The model under review builds one solid part; all positions refer to its coordinate system, in mm. A direction names the side the tool comes from. Give positions to 0.01 mm unless a question says otherwise; leave off trailing zeros. Loops run counter-clockwise (first coordinate to the right, second up) from the corner with the lowest first, then second, coordinate; pieces in that order, holes last. Notation, with made-up numbers: (27, -36) - (73, -36) arc R18 cw to (73, -23) - close; hole circle Ø10 at (33.5, -16). An arc over 180 degrees is marked (long way). Return JSON: item names as keys, results as strings. Group by question number.
```python
from build123d import *

# Parameters (mm, degrees)
EXTRUDE_START       = 2
SKETCH_3_R          = 40.25
SKETCH_3_R_2        = 1.6
SKETCH_3_R_3        = 17.5
EXTRUDE_1_DEPTH     = 3
SKETCH_3_4_R        = 17.5
SKETCH_3_4_R_2      = 2.1
EXTRUDE_3_DEPTH     = 2.5
CHAMFER_1_SIZE      = 3
CHAMFER_4_SIZE      = 2.5
SKETCH_4_R          = 40.25
SKETCH_4_R_2        = 33
SKETCH_4_R_3        = 1.6
EXTRUDE_4_DEPTH     = 2
CUT_EXTRUDE_START   = -13
SKETCH_4_4_R        = 40.25
SKETCH_4_4_R_2      = 33
SKETCH_4_4_R_3      = 1.6
CUT_EXTRUDE_4_DEPTH = 12
CHAMFER_5_SIZE      = 2
CHAMFER_8_SIZE      = 2
SKETCH_5_R          = 1.6
EXTRUDE_5_DEPTH     = 6.5


# Some blends are built 0.0001 mm under size
with BuildPart() as part:
    # 草图3 → 凸台-拉伸1 (new body)
    with BuildSketch(Plane(origin=(0, 0, 0), x_dir=(1, 0, 0), z_dir=(0, 1, 0)).offset(EXTRUDE_START)):
        with Locations(Location((-0.44726781, 0.687620087, 0), (0, 0, 270))):
            Circle(SKETCH_3_R)
        with Locations(Location((-15.663111428, 34.961926834, 0), (0, 0, 270))):
            Circle(SKETCH_3_R_2, mode=Mode.SUBTRACT)
        with Locations(Location((9.927819446, 36.723818061, 0), (0, 0, 270))):
            Circle(SKETCH_3_R_2, mode=Mode.SUBTRACT)
        with Locations(Location((30.664131688, 21.623971758, 0), (0, 0, 270))):
            Circle(SKETCH_3_R_2, mode=Mode.SUBTRACT)
        with Locations(Location((36.843074339, -3.272226173, 0), (0, 0, 270))):
            Circle(SKETCH_3_R_2, mode=Mode.SUBTRACT)
        with Locations(Location((25.573451463, -26.315568031, 0), (0, 0, 270))):
            Circle(SKETCH_3_R_2, mode=Mode.SUBTRACT)
        with Locations(Location((2.128444851, -36.723818061, 0), (0, 0, 270))):
            Circle(SKETCH_3_R_2, mode=Mode.SUBTRACT)
        with Locations(Location((-22.521766341, -29.6268404, 0), (0, 0, 270))):
            Circle(SKETCH_3_R_2, mode=Mode.SUBTRACT)
        with Locations(Location((-36.843074339, -8.34538977, 0), (0, 0, 270))):
            Circle(SKETCH_3_R_2, mode=Mode.SUBTRACT)
        with Locations(Location((-34.134379969, 17.162706563, 0), (0, 0, 270))):
            Circle(SKETCH_3_R_2, mode=Mode.SUBTRACT)
        with Locations(Location((-0.44726781, 0.687620087, 0), (0, 0, 270))):
            Circle(SKETCH_3_R_3, mode=Mode.SUBTRACT)
    extrude(amount=EXTRUDE_1_DEPTH)

    # 草图3<4> → 凸台-拉伸3 (add)
    with BuildSketch(Plane(origin=(0, 0, 0), x_dir=(1, 0, 0), z_dir=(0, 1, 0))):
        with Locations(Location((-0.44726781, 0.687620087, 0), (0, 0, 270))):
            Circle(SKETCH_3_4_R)
        with Locations(Location((-1.271495861, 12.659280294, 0), (0, 0, 270))):
            Circle(SKETCH_3_4_R_2, mode=Mode.SUBTRACT)
        with Locations(Location((9.508380029, 7.387252622, 0), (0, 0, 270))):
            Circle(SKETCH_3_4_R_2, mode=Mode.SUBTRACT)
        with Locations(Location((10.332608081, -4.584407586, 0), (0, 0, 270))):
            Circle(SKETCH_3_4_R_2, mode=Mode.SUBTRACT)
        with Locations(Location((0.376960242, -11.28404012, 0), (0, 0, 270))):
            Circle(SKETCH_3_4_R_2, mode=Mode.SUBTRACT)
        with Locations(Location((-10.402915649, -6.012012448, 0), (0, 0, 270))):
            Circle(SKETCH_3_4_R_2, mode=Mode.SUBTRACT)
        with Locations(Location((-11.227143701, 5.959647759, 0), (0, 0, 270))):
            Circle(SKETCH_3_4_R_2, mode=Mode.SUBTRACT)
    extrude(amount=EXTRUDE_3_DEPTH)

    # 倒角1
    # the kernel refuses this chamfer: 3 mm, written as the material it adds along each edge
    with BuildSketch(Plane(origin=(-0.44726781, 2, -0.687620087), x_dir=(0, 0, 1), z_dir=(-1, 0, 0))) as chamfer_1_piece_1_section:
        Polygon((17.5 + CHAMFER_1_SIZE, 0), (17.5, -CHAMFER_1_SIZE), (17.5, 0), align=None)
    chamfer_1_piece_1 = revolve(axis=Axis((-0.44726781, 2, -0.687620087), (0, 1, 0)), mode=Mode.PRIVATE)
    chamfer_1_piece_1 = split(chamfer_1_piece_1, bisect_by=Plane(origin=(-0.44726781, 0, -20.17366548), z_dir=(0, 1, 0)), keep=Keep.TOP, mode=Mode.PRIVATE)
    add(chamfer_1_piece_1)

    # 倒角4
    chamfer_4_edges = [part.edges().sort_by_distance(p)[0] for p in [
        (-0.44726781, 5, -18.187620087),
    ]]
    chamfer(chamfer_4_edges, length=CHAMFER_4_SIZE - 0.0001)  # a hair under: the kernel refuses the full size

    # 草图4 → 凸台-拉伸4 (add)
    with BuildSketch(Plane(origin=(0, 5, 0), x_dir=(1, 0, 0), z_dir=(0, 1, 0))):
        with Locations(Location((-0.44726781, 0.687620087, 0), (0, 0, 270))):
            Circle(SKETCH_4_R)
        with Locations(Location((-0.44726781, 0.687620087, 0), (0, 0, 270))):
            Circle(SKETCH_4_R_2, mode=Mode.SUBTRACT)
        with Locations(Location((-36.843074339, -8.34538977, 0), (0, 0, 270))):
            Circle(SKETCH_4_R_3, mode=Mode.SUBTRACT)
        with Locations(Location((-22.521766341, -29.6268404, 0), (0, 0, 270))):
            Circle(SKETCH_4_R_3, mode=Mode.SUBTRACT)
        with Locations(Location((2.128444851, -36.723818061, 0), (0, 0, 270))):
            Circle(SKETCH_4_R_3, mode=Mode.SUBTRACT)
        with Locations(Location((25.573451463, -26.315568031, 0), (0, 0, 270))):
            Circle(SKETCH_4_R_3, mode=Mode.SUBTRACT)
        with Locations(Location((36.843074339, -3.272226173, 0), (0, 0, 270))):
            Circle(SKETCH_4_R_3, mode=Mode.SUBTRACT)
        with Locations(Location((30.664131688, 21.623971758, 0), (0, 0, 270))):
            Circle(SKETCH_4_R_3, mode=Mode.SUBTRACT)
        with Locations(Location((9.927819446, 36.723818061, 0), (0, 0, 270))):
            Circle(SKETCH_4_R_3, mode=Mode.SUBTRACT)
        with Locations(Location((-15.663111428, 34.961926834, 0), (0, 0, 270))):
            Circle(SKETCH_4_R_3, mode=Mode.SUBTRACT)
        with Locations(Location((-34.134379969, 17.162706563, 0), (0, 0, 270))):
            Circle(SKETCH_4_R_3, mode=Mode.SUBTRACT)
    extrude(amount=EXTRUDE_4_DEPTH)

    # 草图4<4> → 切除-拉伸4 (cut)
    with BuildSketch(Plane(origin=(0, 5, 0), x_dir=(1, 0, 0), z_dir=(0, 1, 0)).offset(CUT_EXTRUDE_START)):
        with Locations(Location((-0.44726781, 0.687620087, 0), (0, 0, 270))):
            Circle(SKETCH_4_4_R)
        with Locations(Location((-0.44726781, 0.687620087, 0), (0, 0, 270))):
            Circle(SKETCH_4_4_R_2, mode=Mode.SUBTRACT)
        with Locations(Location((-36.843074339, -8.34538977, 0), (0, 0, 270))):
            Circle(SKETCH_4_4_R_3, mode=Mode.SUBTRACT)
        with Locations(Location((-22.521766341, -29.6268404, 0), (0, 0, 270))):
            Circle(SKETCH_4_4_R_3, mode=Mode.SUBTRACT)
        with Locations(Location((2.128444851, -36.723818061, 0), (0, 0, 270))):
            Circle(SKETCH_4_4_R_3, mode=Mode.SUBTRACT)
        with Locations(Location((25.573451463, -26.315568031, 0), (0, 0, 270))):
            Circle(SKETCH_4_4_R_3, mode=Mode.SUBTRACT)
        with Locations(Location((36.843074339, -3.272226173, 0), (0, 0, 270))):
            Circle(SKETCH_4_4_R_3, mode=Mode.SUBTRACT)
        with Locations(Location((30.664131688, 21.623971758, 0), (0, 0, 270))):
            Circle(SKETCH_4_4_R_3, mode=Mode.SUBTRACT)
        with Locations(Location((9.927819446, 36.723818061, 0), (0, 0, 270))):
            Circle(SKETCH_4_4_R_3, mode=Mode.SUBTRACT)
        with Locations(Location((-15.663111428, 34.961926834, 0), (0, 0, 270))):
            Circle(SKETCH_4_4_R_3, mode=Mode.SUBTRACT)
        with Locations(Location((-34.134379969, 17.162706563, 0), (0, 0, 270))):
            Circle(SKETCH_4_4_R_3, mode=Mode.SUBTRACT)
    extrude(amount=CUT_EXTRUDE_4_DEPTH, mode=Mode.SUBTRACT)

    # 倒角5
    chamfer_5_edges = [part.edges().sort_by_distance(p)[0] for p in [
        (-0.44726781, 5, -33.687620087),
    ]]
    chamfer(chamfer_5_edges, length=CHAMFER_5_SIZE - 0.0001)  # a hair under: the kernel refuses the full size

    # 倒角8
    chamfer_8_edges = [part.edges().sort_by_distance(p)[0] for p in [
        (-0.44726781, 2, -33.687620087),
    ]]
    chamfer(chamfer_8_edges, length=CHAMFER_8_SIZE - 0.0001)  # a hair under: the kernel refuses the full size

    # 草图5 → 凸台-拉伸5 (add)
    with BuildSketch(Plane(origin=(0, 7, 0), x_dir=(1, 0, 0), z_dir=(0, 1, 0))):
        with Locations(Location((9.927819446, 36.723818061, 0), (0, 0, 270))):
            Circle(SKETCH_5_R)
        with BuildLine():
            Line((21.54973721, -26.536115332), (20.292765494, -24.980473308))
            ThreePointArc((20.292765494, -24.980473308), (12.942674574, -29.47376985), (4.680081209, -31.911617512))
            Line((4.680081209, -31.911617512), (4.990829634, -33.887328882))
            ThreePointArc((4.990829634, -33.887328882), (13.754186234, -31.301732877), (21.54973721, -26.536115332))
        make_face()
        with BuildLine():
            Line((12.130676139, 33.34945295), (11.411936485, 31.483062501))
            ThreePointArc((11.411936485, 31.483062501), (18.978290897, 27.364345315), (25.220825585, 21.427653391))
            Line((25.220825585, 21.427653391), (26.776467609, 22.684625106))
            ThreePointArc((26.776467609, 22.684625106), (20.155597485, 28.981116541), (12.130676139, 33.34945295))
        make_face()
        with BuildLine():
            Line((-35.022216779, -4.750477357), (-33.046505409, -4.439728932))
            ThreePointArc((-33.046505409, -4.439728932), (-33.262768901, 4.172284796), (-31.242710224, 12.546824382))
            Line((-31.242710224, 12.546824382), (-33.109100673, 13.265564036))
            ThreePointArc((-33.109100673, 13.265564036), (-35.251587149, 4.383476596), (-35.022216779, -4.750477357))
        make_face()
    extrude(amount=EXTRUDE_5_DEPTH)


with BuildPart() as extrude_5_kept_piece:
    # of the separate pieces the step leaves, the one the design keeps (extrude_5_pieces_kept)
    add(part.part.solids().sort_by_distance((-0.44726781, 3.9999, 32.312379913))[0])


solid = extrude_5_kept_piece.part
```
1) For pin 1 Ø4 at (x, z) = (-36.84, 8.35) entering from -Y; pin 2 Ø5 at (x, z) = (10.33, 4.58) entering from +Y; pin 3 Ø4 at (x, z) = (13, 26.5) entering from +Y; pin 4 Ø2.5 at (x, z) = (0.38, 11.28) entering from -Y, all flat-tipped, find the tip position at first contact; note any pin that passes through.
2) Draft analysis for pull direction X (two halves, no side actions). For faces 5 (the face through (19, 13.5, -28)), 6 (the face through (2.61, 5.48, 38.25)), 7 (the face through (-34.048, 10.204, 4.597)), state which applies: +X half, -X half, draft (parallel to the pull), parting line (faces both ways), or undercut.
3) We need section A-A, the plane y = 11.25. Write out the cut boundary in (x, z), plus the area to 3 significant figures.
4) Tool access review of faces 1 (the face through (33, 7, -4)), 2 (the face through (13.64, 10.2, 31.35)), 3 (the face through (-12.266, 1.232, 6.981)), 4 (the face through (3, 4, -34)): name each direction out of +Z, -Z, +X, -X, +Y, -Y from which nothing blocks a thin tool from reaching the whole face with its end or side.
5) To check wall thickness, follow line 1 (Z direction, x = 10.5, y = 1.5); line 2 (Y direction, x = -24.5, z = 10); line 3 (Z direction, x = 16.5, y = 12.5). State the ranges of each line that lie inside material, in increasing order.
Findings:
{
 "1": {"pin 1": "stops at y = 4", "pin 2": "stops at y = 2.5", "pin 3": "stops at y = 6.33", "pin 4": "passes through"},
 "2": {"face 5": "draft", "face 6": "undercut", "face 7": "+X half"},
 "3": {"outline": "(-35.02, 4.75) arc R35 ccw to (-33.11, -13.27) - (-31.24, -12.55) arc R33 cw to (-33.05, 4.44) - close; (4.68, 31.91) arc R33 cw to (20.29, 24.98) - (21.55, 26.54) arc R35 ccw to (4.99, 33.89) - close; (11.41, -31.48) - (12.13, -33.35) arc R35 ccw to (26.78, -22.68) - (25.22, -21.43) arc R33 cw to start", "area": "107 mm^2"},
 "4": {"face 1": "+Y", "face 2": "+Z, +X, +Y", "face 3": "+Y, -Y", "face 4": "-Y"},
 "5": {"line 1": "z = -17.43 to -9.24, -5.54 to 2.49, 6.68 to 16.05", "line 2": "y = 2 to 5", "line 3": "z = -31.31 to -29, 27.63 to 29.94"}
}
